Design review of the part built by this model. Coordinates are the model's own, in mm. A direction names the side the tool comes from. Coordinates: 2 decimals unless noted, no trailing zeros. Loops run counter-clockwise (first coordinate to the right, second up) from the corner with the lowest first, then second, coordinate; pieces in that order, holes last. Notation, with made-up numbers: (-9, -19) - (11, -19) arc R15 cw to (11, -9) - close; hole circle Ø4 at (68, 55.25). An arc over 180 degrees is marked (long way). Answer in a Markdown table with one row per item. Add a question column.
(1) Clearance check with flat-ended pins moving along their axes: pin 1 (3 mm diameter, centred on x = 0, z = -20, fed in from +Y); pin 2 (2 mm diameter, centred on x = -1.5, y = 7.5, fed in from +Z); pin 3 (1 mm diameter, centred on x = 2, y = 38.5, fed in from -Z); pin 4 (6 mm diameter, centred on x = 1.5, y = 34.5, fed in from -Z). State where each tip first meets the part, or that it passes through.
(2) We need section A-A, the plane z = -16. Write out the cut boundary in (x, y).
(3) We need section D-D, the plane x = -2.5. Write out the cut boundary in (y, z), plus the area to 3 significant figures.
(4) To check wall thickness, follow L1, parallel to X at y = 2.65, z = -20; L2, parallel to Y at x = 3, z = -22; L3, parallel to Y at x = -4, z = -3. State the ranges of each line that lie inside material, in increasing order. Write a range as [from, to].
(5) The part is to be moulded in two halves that separate along X. For faces 4 (the face through (0.08, 40.1, -13.36)), 5 (the face through (0, 43, -26)), 6 (the face through (-2, 2, 0)), say which applies: released by +X, released by -X, zero draft, split by the parting line, or undercut.
(6) We need section C-C, the plane z = 1.5. Write out the cut boundary in (x, y), plus the area to 3 significant figures.
(7) For faces 1 (the face through (0, 22, -12.5)), 2 (the face through (6, 22, -10)), 3 (the face through (0, 26, -7.5)), list the 3-axis set-ups (+Z, -Z, +X, -X, +Y, -Y) from which the entire face can be reached by the end or side of a thin tool; tool diameter is ignored.
(8) We need section B-B, the plane x = 0. Write out the cut boundary in (y, z), plus the area to 3 significant figures.
from build123d import *

# Parameters (mm, degrees)
SKETCH1_R           = 2
BOSS_EXTRUDE1_DEPTH = 4
SKETCH2_W           = 12
SKETCH2_H           = 5
BOSS_EXTRUDE2_DEPTH = 37
SKETCH3_R           = 2
SKETCH3_W           = 12
SKETCH3_H           = 5
BOSS_EXTRUDE3_DEPTH = 4
FILLET1_R           = 3


with BuildPart() as part:
    # Sketch1 → Boss-Extrude1 (new body)
    with BuildSketch(Plane(origin=(0, 0, 0), x_dir=(1, 0, 0), z_dir=(0, 1, 0))):
        with BuildLine():
            ThreePointArc((6, 20), (0, 26), (-6, 20))
            Line((-6, 20), (-6, 0))
            ThreePointArc((-6, 0), (0, -6), (6, 0))
            Line((6, 0), (6, 20))
        make_face()
        with Locations(Location((0, 20, 0), (0, 0, 270))):
            Circle(SKETCH1_R, mode=Mode.SUBTRACT)
        with Locations(Location((0, 0, 0), (0, 0, 270))):
            Circle(SKETCH1_R, mode=Mode.SUBTRACT)
    extrude(amount=BOSS_EXTRUDE1_DEPTH)

    # Sketch2 → Boss-Extrude2 (add)
    with BuildSketch(Plane(origin=(0, 4, 0), x_dir=(1, 0, 0), z_dir=(0, 1, 0))):
        with Locations((0, 10)):
            Rectangle(SKETCH2_W, SKETCH2_H)
    extrude(amount=BOSS_EXTRUDE2_DEPTH)

    # Sketch3 → Boss-Extrude3 (add)
    # profile 1 of 2: a face of its own
    with BuildSketch(Plane(origin=(0, 41, 0), x_dir=(1, 0, 0), z_dir=(0, 1, 0))):
        with BuildLine():
            Line((6, 12.5), (6, 20))
            ThreePointArc((6, 20), (0, 26), (-6, 20))
            Line((-6, 20), (-6, 12.5))
            Line((-6, 12.5), (6, 12.5))
        make_face()
        with Locations(Location((0, 20, 0), (0, 0, 270))):
            Circle(SKETCH3_R, mode=Mode.SUBTRACT)
    # profile 2 of 2: a face of its own
    with BuildSketch(Plane(origin=(0, 41, 0), x_dir=(1, 0, 0), z_dir=(0, 1, 0))):
        with Locations((0, 10)):
            Rectangle(SKETCH3_W, SKETCH3_H)
    extrude(amount=BOSS_EXTRUDE3_DEPTH)

    # Fillet1
    fillet1_edges = [part.edges().sort_by_distance(p)[0] for p in [
        (0, 4, -12.5),
        (0, 41, -12.5),
        (0, 4, -7.5),
    ]]
    fillet(fillet1_edges, radius=FILLET1_R)


solid = part.part
Responses:
| question | item | result |
|---|---|---|
| 1 | pin 1 | passes through |
| 1 | pin 2 | stops at z = -7.46 |
| 1 | pin 3 | stops at z = -12.67 |
| 1 | pin 4 | stops at z = -12.5 |
| 2 | outline | (-6, 0) - (6, 0) - (6, 4) - (-6, 4) - close; (-6, 41) - (6, 41) - (6, 45) - (-6, 45) - close |
| 3 | outline | (0, -25.45) - (4, -25.45) - (4, -15.5) arc R3 cw to (7, -12.5) - (38, -12.5) arc R3 cw to (41, -15.5) - (41, -25.45) - (45, -25.45) - (45, -7.5) - (7, -7.5) arc R3 cw to (4, -4.5) - (4, 5.45) - (0, 5.45) - close |
| 3 | area | 386 mm2 |
| 4 | L1 | x = [-6, -2], [2, 6] |
| 4 | L2 | y = [0, 4], [41, 45] |
| 4 | L3 | y = [0, 4] |
| 5 | face 4 | zero draft |
| 5 | face 5 | split by the parting line |
| 5 | face 6 | undercut |
| 6 | outline | (-5.81, 0) - (-1.32, 0) - (-1.32, 4) - (-5.81, 4) - close; (1.32, 0) - (5.81, 0) - (5.81, 4) - (1.32, 4) - close |
| 6 | area | 35.9 mm2 |
| 7 | face 1 | -Z, +X, -X |
| 7 | face 2 | +Z, -Z, +X, +Y, -Y |
| 7 | face 3 | +Z, +X, -X, +Y |
| 8 | outline | (0, -26) - (4, -26) - (4, -22) - (0, -22) - close; (0, -18) - (4, -18) - (4, -15.5) arc R3 cw to (7, -12.5) - (38, -12.5) arc R3 cw to (41, -15.5) - (41, -18) - (45, -18) - (45, -7.5) - (7, -7.5) arc R3 cw to (4, -4.5) - (4, -2) - (0, -2) - close; (0, 2) - (4, 2) - (4, 6) - (0, 6) - close; (41, -26) - (45, -26) - (45, -22) - (41, -22) - close |
| 8 | area | 345 mm2 |
